Read the model definition and answer for the solid it produces. Units are mm, in the model's axes. Coordinates: 2 decimals unless noted, no trailing zeros. Loops run counter-clockwise (first coordinate to the right, second up) from the corner with the lowest first, then second, coordinate; pieces in that order, holes last. Notation, with made-up numbers: (-24, 63) -> (15, 63) arc R14 ccw to (15, 75) -> close; hole circle Ø10 at (-9, 52). An arc over 180 degrees is marked (long way). Answer as a JSON object with one key per item and string values. Group by question number.
Q1. The part is cut by section C-C on x = 10. Write down the section's boundary in (y, z), and give its area (3 significant figures).
Q2. The part is cut by section B-B on x = 0. Write down the section's boundary in (y, z).
Q3. Each of these flat-tipped pins is pushed along its axis until it touches: P1, Ø6, axis at x = -10, y = 5.5, coming from the +Z side; P2, Ø1, axis at x = -13, z = 20.5, coming from the +Y side; P3, Ø4, axis at x = -10, y = 0, coming from the -Z side; P4, Ø2, axis at x = 13.5, z = 56.5, coming from the +Y side. Where does it stop, or does it pass through?
Q4. Straight lines are drawn through the part: line 1 along Y through (x, z) = (18, -86.5); line 2 along Y through (x, z) = (-2, 96); line 3 along X through (y, z) = (7.75, 21). For each, find the intervals that lie inside material, in ascending order. Write a range as [from, to].
Q5. The part is cut by section D-D on z = 5.5. State how many separate pieces and enclosed holes the cut face has, and give its area (3 significant figures).
Q6. The part is cut by section A-A on y = 0. Write down the section's boundary in (x, z).
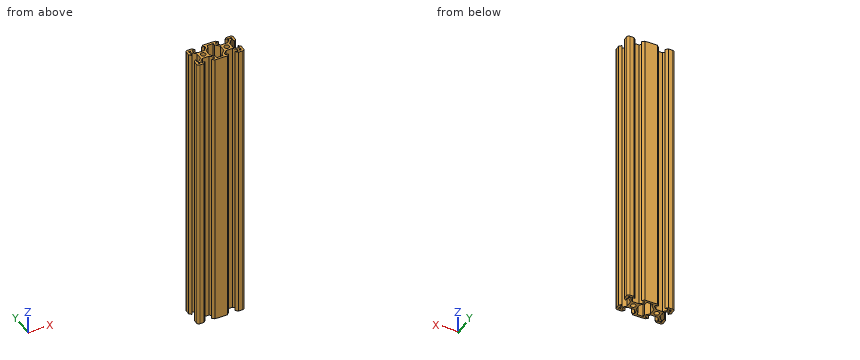
from build123d import *

# Parameters (mm, degrees)
ESQUISSE1_R        = 2.1
BOSS_EXTRU_1_DEPTH = 125


with BuildPart() as part:
    # Esquisse1 → Boss.-Extru.1 (new, symmetric)
    with BuildSketch(Plane.XY):
        with BuildLine():
            Line((-10, 3.900660172), (-12.84, 3.900660172))
            Line((-12.84, 3.900660172), (-15.499339828, 6.56))
            Line((-15.499339828, 6.56), (-15.499339828, 8.2))
            Line((-15.499339828, 8.2), (-12.84, 8.2))
            Line((-12.84, 8.2), (-14.64, 10))
            Line((-14.64, 10), (-18.2, 10))
            ThreePointArc((-18.2, 10), (-19.472792206, 9.472792206), (-20, 8.2))
            Line((-20, 8.2), (-20, 4.64))
            Line((-20, 4.64), (-18.2, 2.84))
            Line((-18.2, 2.84), (-18.2, 5.499339828))
            Line((-18.2, 5.499339828), (-16.56, 5.499339828))
            Line((-16.56, 5.499339828), (-13.900660172, 2.84))
            Line((-13.900660172, 2.84), (-13.900660172, 0))
            Line((-13.900660172, 0), (-13.900660172, -2.84))
            Line((-13.900660172, -2.84), (-16.56, -5.499339828))
            Line((-16.56, -5.499339828), (-18.2, -5.499339828))
            Line((-18.2, -5.499339828), (-18.2, -2.84))
            Line((-18.2, -2.84), (-20, -4.64))
            Line((-20, -4.64), (-20, -8.2))
            ThreePointArc((-20, -8.2), (-19.472792206, -9.472792206), (-18.2, -10))
            Line((-18.2, -10), (-14.64, -10))
            Line((-14.64, -10), (-12.84, -8.2))
            Line((-12.84, -8.2), (-15.499339828, -8.2))
            Line((-15.499339828, -8.2), (-15.499339828, -6.56))
            Line((-15.499339828, -6.56), (-12.84, -3.900660172))
            Line((-12.84, -3.900660172), (-10, -3.900660172))
            Line((-10, -3.900660172), (-7.16, -3.900660172))
            Line((-7.16, -3.900660172), (-4.500660172, -6.56))
            Line((-4.500660172, -6.56), (-4.500660172, -8.2))
            Line((-4.500660172, -8.2), (-7.16, -8.2))
            Line((-7.16, -8.2), (-5.36, -10))
            Line((-5.36, -10), (5.36, -10))
            Line((5.36, -10), (7.16, -8.2))
            Line((7.16, -8.2), (4.500660172, -8.2))
            Line((4.500660172, -8.2), (4.500660172, -6.56))
            Line((4.500660172, -6.56), (7.16, -3.900660172))
            Line((7.16, -3.900660172), (10, -3.900660172))
            Line((10, -3.900660172), (12.84, -3.900660172))
            Line((12.84, -3.900660172), (15.499339828, -6.56))
            Line((15.499339828, -6.56), (15.499339828, -8.2))
            Line((15.499339828, -8.2), (12.84, -8.2))
            Line((12.84, -8.2), (14.64, -10))
            Line((14.64, -10), (18.2, -10))
            ThreePointArc((18.2, -10), (19.472792206, -9.472792206), (20, -8.2))
            Line((20, -8.2), (20, -4.64))
            Line((20, -4.64), (18.2, -2.84))
            Line((18.2, -2.84), (18.2, -5.499339828))
            Line((18.2, -5.499339828), (16.56, -5.499339828))
            Line((16.56, -5.499339828), (13.900660172, -2.84))
            Line((13.900660172, -2.84), (13.900660172, 0))
            Line((13.900660172, 0), (13.900660172, 2.84))
            Line((13.900660172, 2.84), (16.56, 5.499339828))
            Line((16.56, 5.499339828), (18.2, 5.499339828))
            Line((18.2, 5.499339828), (18.2, 2.84))
            Line((18.2, 2.84), (20, 4.64))
            Line((20, 4.64), (20, 8.2))
            ThreePointArc((20, 8.2), (19.472792206, 9.472792206), (18.2, 10))
            Line((18.2, 10), (14.64, 10))
            Line((14.64, 10), (12.84, 8.2))
            Line((12.84, 8.2), (15.499339828, 8.2))
            Line((15.499339828, 8.2), (15.499339828, 6.56))
            Line((15.499339828, 6.56), (12.84, 3.900660172))
            Line((12.84, 3.900660172), (10, 3.900660172))
            Line((10, 3.900660172), (7.16, 3.900660172))
            Line((7.16, 3.900660172), (4.500660172, 6.56))
            Line((4.500660172, 6.56), (4.500660172, 8.2))
            Line((4.500660172, 8.2), (7.16, 8.2))
            Line((7.16, 8.2), (5.36, 10))
            Line((5.36, 10), (-5.36, 10))
            Line((-5.36, 10), (-7.16, 8.2))
            Line((-7.16, 8.2), (-4.500660172, 8.2))
            Line((-4.500660172, 8.2), (-4.500660172, 6.56))
            Line((-4.500660172, 6.56), (-7.16, 3.900660172))
            Line((-7.16, 3.900660172), (-10, 3.900660172))
        make_face()
        with Locations((-10, 0)):
            Circle(ESQUISSE1_R, mode=Mode.SUBTRACT)
        with Locations(Location((10, 0, 0), (0, 0, 180))):
            Circle(ESQUISSE1_R, mode=Mode.SUBTRACT)
        Polygon((-2.7, 8.2), (-2.7, 6.239339828), (-6.099339828, 2.84), (-6.099339828, -2.84), (-2.7, -6.239339828), (-2.7, -8.2), (2.7, -8.2), (2.7, -6.239339828), (6.099339828, -2.84), (6.099339828, 2.84), (2.7, 6.239339828), (2.7, 8.2), align=None, mode=Mode.SUBTRACT)
        Polygon((-18.2, 8.2), (-18.2, 6.569339828), (-17.63, 6.569339828), (-16.569339828, 7.63), (-16.569339828, 8.2), align=None, mode=Mode.SUBTRACT)
        Polygon((-18.2, -6.569339828), (-17.63, -6.569339828), (-16.569339828, -7.63), (-16.569339828, -8.2), (-18.2, -8.2), align=None, mode=Mode.SUBTRACT)
        Polygon((18.2, 6.569339828), (17.63, 6.569339828), (16.569339828, 7.63), (16.569339828, 8.2), (18.2, 8.2), align=None, mode=Mode.SUBTRACT)
        Polygon((18.2, -6.569339828), (17.63, -6.569339828), (16.569339828, -7.63), (16.569339828, -8.2), (18.2, -8.2), align=None, mode=Mode.SUBTRACT)
    extrude(amount=BOSS_EXTRU_1_DEPTH, both=True)


solid = part.part
Final values:
{
 "1": {"outline": "(-3.9, -125) -> (-2.1, -125) -> (-2.1, 125) -> (-3.9, 125) -> close; (2.1, -125) -> (3.9, -125) -> (3.9, 125) -> (2.1, 125) -> close", "area": "900 mm2"},
 "2": {"outline": "(-10, -125) -> (-8.2, -125) -> (-8.2, 125) -> (-10, 125) -> close; (8.2, -125) -> (10, -125) -> (10, 125) -> (8.2, 125) -> close"},
 "3": {"P1": "stops at z = 125", "P2": "stops at y = 8.86", "P3": "passes through", "P4": "stops at y = 9.86"},
 "4": {"line 1": "y = [-10, -8.2], [-6.57, -5.5], [5.5, 6.57], [8.2, 10]", "line 2": "y = [-10, -8.2], [8.2, 10]", "line 3": "x = [-20, -18.2], [-16.57, -15.5], [-4.5, -2.7], [2.7, 4.5], [15.5, 16.57], [18.2, 20]"},
 "5": {"separate pieces": "1", "enclosed holes": "7", "area": "289 mm2"},
 "6": {"outline": "(-13.9, -125) -> (-12.1, -125) -> (-12.1, 125) -> (-13.9, 125) -> close; (-7.9, -125) -> (-6.1, -125) -> (-6.1, 125) -> (-7.9, 125) -> close; (6.1, -125) -> (7.9, -125) -> (7.9, 125) -> (6.1, 125) -> close; (12.1, -125) -> (13.9, -125) -> (13.9, 125) -> (12.1, 125) -> close"}
}
